Job drawing, mm, ordinate dimensions from the low corner. One solid piece. A direction names the side the tool comes from. Round coordinates to 2 decimals unless told otherwise and drop trailing zeros. Order: outer loops, then holes, each group sorted by start corner. A loop starts at its lowest first (then second) coordinate and runs counter-clockwise, first axis right, second up. Notation, with made-up numbers: (15.5, 61) -> (53.5, 61) arc R26 ccw to (53.5, 89) -> close; hole circle Ø7 at (86, -29). An arc over 180 degrees is marked (long way). Answer as a JSON object with one key per item and string values. Group by question number.
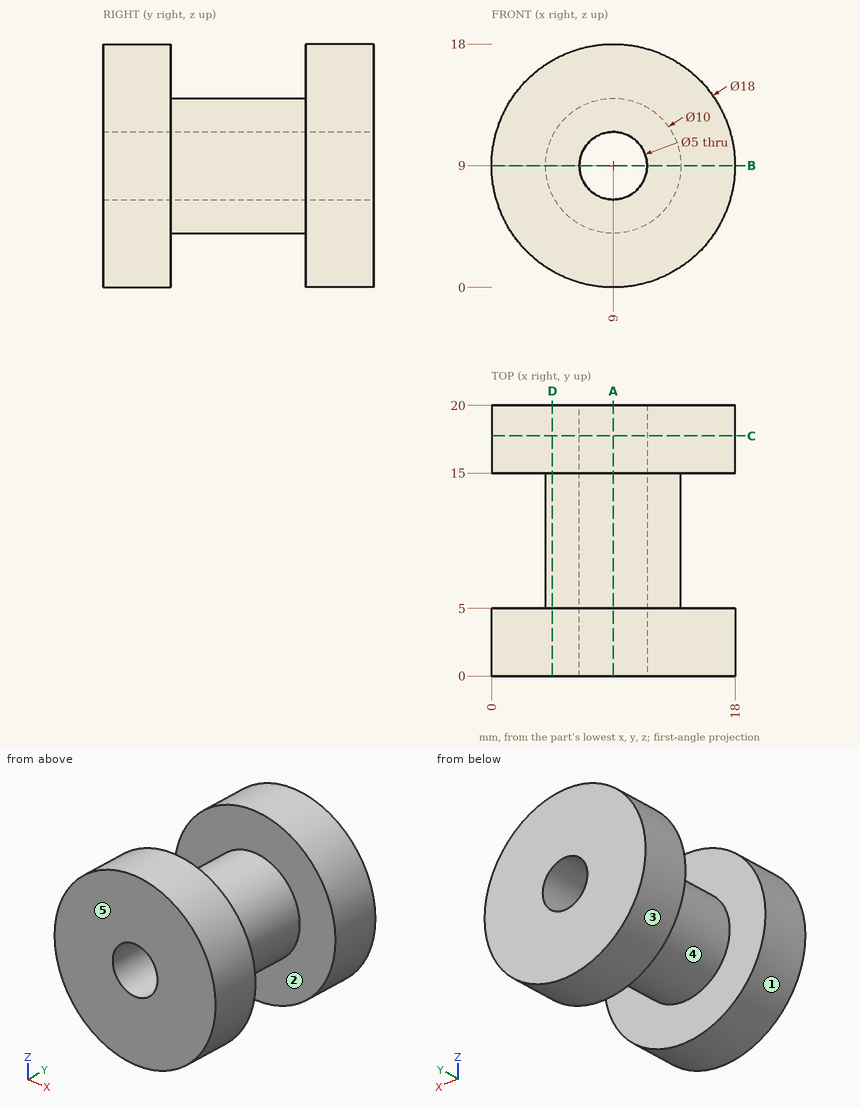
Q1. Two-plate mould, pull along Y, no slides. Class the marked faces 3, 4 and 5: +Y half, -Y half, draft (parallel to the pull), parting line (faces both ways), or undercut.
Q2. Drop flat-ended pins along their axis: pin 1 Ø3 at (x, y) = (15, 10.5) entering from -Z; pin 2 Ø3 at (y, z) = (4, 7) entering from -X; pin 3 Ø1.5 at (x, y) = (13, 8) entering from -Z. Give the stop position or say it passes through.
Q3. Which spindle directions (+Z, -Z, +X, -X, +Y, -Y) get a long thin tool onto all of the face, cutting with end or side? Do the marked faces 1 and 2. Say none if no direction does.
Q4. Band-saw the part on B-B (z = 9). List the corners of the cut face in (x, y).
Q5. Band-saw the part on C-C (y = 17.75). List the corners of the cut face in (x, z).
Q6. Band-saw the part on D-D (x = 4.5). List the corners of the cut face in (y, z), plus the area to 3 significant figures.
Q7. Band-saw the part on A-A (x = 9). List the corners of the cut face in (y, z).
Q8. Wall check: line 1 (Z direction, x = 9, y = 5.25); line 2 (Y direction, x = 8, z = 17); line 3 (Z direction, x = 9, y = 16). Give the ranges that are in metal, low to high. Write a range as [from, to].
Completed:
{
 "1": {"face 3": "draft", "face 4": "undercut", "face 5": "-Y half"},
 "2": {"pin 1": "z = 6.82", "pin 2": "x = 0.01", "pin 3": "z = 5.2"},
 "3": {"face 1": "+Y, -Y", "face 2": "none"},
 "4": {"outline": "(0, 0) -> (6.5, 0) -> (6.5, 20) -> (0, 20) -> (0, 15) -> (4, 15) -> (4, 5) -> (0, 5) -> close; (11.5, 0) -> (18, 0) -> (18, 5) -> (14, 5) -> (14, 15) -> (18, 15) -> (18, 20) -> (11.5, 20) -> close"},
 "5": {"outline": "circle Ø18 at (9, 9); hole circle Ø5 at (9, 9)"},
 "6": {"outline": "(0, 1.21) -> (5, 1.21) -> (5, 6.82) -> (15, 6.82) -> (15, 1.21) -> (20, 1.21) -> (20, 16.79) -> (15, 16.79) -> (15, 11.18) -> (5, 11.18) -> (5, 16.79) -> (0, 16.79) -> close", "area": "199 mm2"},
 "7": {"outline": "(0, 0) -> (5, 0) -> (5, 4) -> (15, 4) -> (15, 0) -> (20, 0) -> (20, 6.5) -> (0, 6.5) -> close; (0, 11.5) -> (20, 11.5) -> (20, 18) -> (15, 18) -> (15, 14) -> (5, 14) -> (5, 18) -> (0, 18) -> close"},
 "8": {"line 1": "[4, 6.5], [11.5, 14]", "line 2": "[0, 5], [15, 20]", "line 3": "[0, 6.5], [11.5, 18]"}
}
